Job drawing, mm, ordinate dimensions from the low corner. One solid piece. Coordinates: 2 decimals unless noted, no trailing zeros. Loops run counter-clockwise (first coordinate to the right, second up) from the corner with the lowest first, then second, coordinate; pieces in that order, holes last. Notation, with made-up numbers: (70.25, 36) - (79.25, 36) arc R15 cw to (79.25, 52) - close; hole circle Ø11 at (28, -7). An arc over 180 degrees is marked (long way). Use a Markdown table: item, result. Add a question column.
1. Band-saw the part on D-D, the plane z = 53. Give the cut face in (x, y) (3 decimals).
2. Band-saw the part on B-B, the plane y = 9.5. Give the cut face in (x, z).
3. Drop flat-ended pins along their axis: pin 1 (22 mm diameter, centred on x = 68.5, z = 20, fed in from +Y); pin 2 (2 mm diameter, centred on y = 3.5, z = 39.5, fed in from -X) (3 decimals); pin 3 (1.5 mm diameter, centred on x = 66, y = 5, fed in from +Z); pin 4 (5.5 mm diameter, centred on y = 8, z = 52.5, fed in from +X). Give the stop position or say it passes through.
4. Band-saw the part on A-A, the plane z = 8. Give the cut face in (x, y) (3 decimals).
5. Band-saw the part on C-C, the plane x = 55.5. Give the cut face in (y, z), plus the area to 3 significant figures.
6. Wall check: probe 1 along Y at (x, z) = (111, 55); probe 2 along X at (y, z) = (9.5, 69); probe 3 along X at (y, z) = (2.5, 37.5) (3 decimals). Give the ranges that are in metal, low to high. Write a range as [from, to].
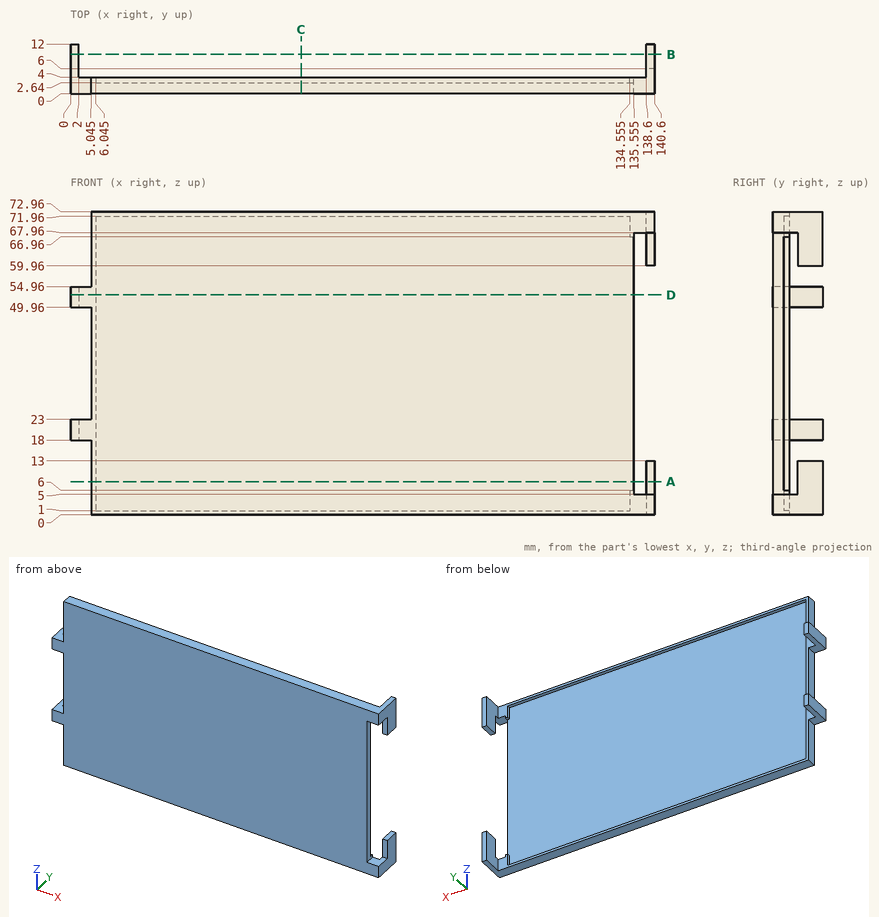
Geometry check:
| question | item | result |
|---|---|---|
| 1 | outline | (0, 0) - (135.555, 0) - (135.555, 2.64) - (6.045, 2.64) - (6.045, 4) - (2, 4) - (2, 12) - (0, 12) - close |
| 2 | outline | (0, 18) - (2, 18) - (2, 23) - (0, 23) - close; (0, 49.96) - (2, 49.96) - (2, 54.96) - (0, 54.96) - close; (138.6, 0) - (140.6, 0) - (140.6, 13) - (138.6, 13) - close; (138.6, 59.96) - (140.6, 59.96) - (140.6, 72.96) - (138.6, 72.96) - close |
| 3 | pin 1 | stops at y = 2.64 |
| 3 | pin 2 | stops at x = 5.045 |
| 3 | pin 3 | passes through |
| 3 | pin 4 | stops at x = 2 |
| 4 | outline | (5.045, 0) - (135.555, 0) - (135.555, 2.64) - (6.045, 2.64) - (6.045, 4) - (5.045, 4) - close; (138.6, 6) - (140.6, 6) - (140.6, 12) - (138.6, 12) - close |
| 5 | outline | (0, 0) - (4, 0) - (4, 1) - (2.64, 1) - (2.64, 71.96) - (4, 71.96) - (4, 72.96) - (0, 72.96) - close |
| 5 | area | 195 mm^2 |
| 6 | probe 1 | y = [0, 2.64] |
| 6 | probe 2 | x = [138.6, 140.6] |
| 6 | probe 3 | x = [5.045, 135.555] |
